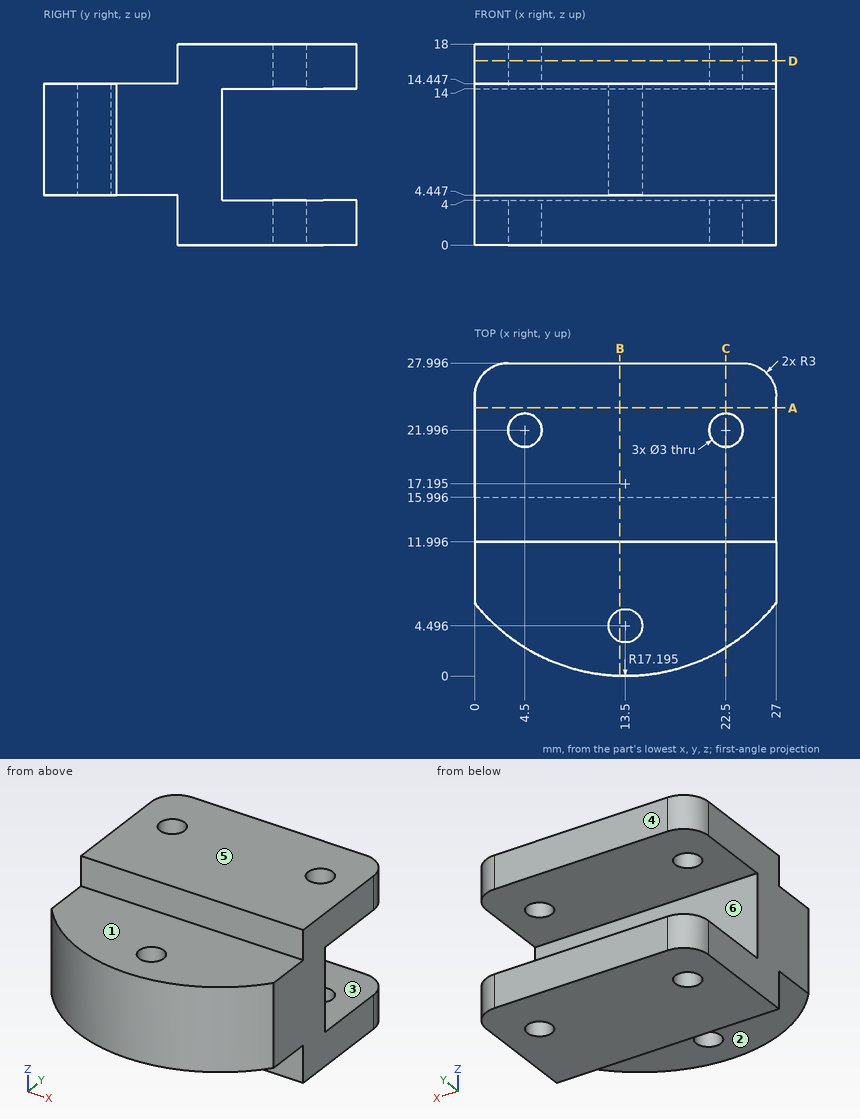
Job drawing, mm, ordinate dimensions from the low corner. One solid piece. A direction names the side the tool comes from. Coordinates: 2 decimals unless noted, no trailing zeros. Write each loop counter-clockwise with the first axis right and the second up, starting at its lowest first coordinate (ties: lowest second). Pieces come first, ordered by that corner, then holes. Notation, with made-up numbers: (15, -8) -> (49, -8) arc R14 cw to (49, 17) -> close; hole circle Ø6 at (50, 32.25). An arc over 180 degrees is marked (long way). Use CSV: the item, a comma, the result in double quotes. Start each with the question number.
Item 1: Band-saw the part on D-D, the plane z = 16.5. Write the cut outline in (x, y).
Item 2: Drop flat-ended pins along their axis: P1, Ø4, axis at y = 4.5, z = 8.5, coming from the +X side (1 decimal); P2, Ø5, axis at x = 4.5, y = 22, coming from the +Z side; P3, Ø1.8, axis at x = 7, z = 16, coming from the -Y side; P4, Ø6, axis at x = 13.5, y = 7.5, coming from the -Z side. Give the stop position or say it passes through.
Item 3: Band-saw the part on A-A, the plane y = 24. Write the cut outline in (x, z).
Item 4: Wall check: probe 1 along Z at (x, y) = (15.5, 22); probe 2 along Y at (x, z) = (22.5, 2); probe 3 along Y at (x, z) = (13.5, 11). Give the ranges that are in metal, low to high.
Item 5: Two-plate mould, pull along Z, no slides. Class the marked faces 4, 5 and 6: +Z half, -Z half, draft (parallel to the pull), parting line (faces both ways), or undercut.
Item 6: Tool access for the marked faces 1, 2 and 3: list every direction of +Z, -Z, +X, -X, +Y, -Y with a clear straight run to the whole face (end or side of a thin tool).
Item 7: Band-saw the part on B-B, the plane x = 13. Write the cut outline in (y, z).
Item 8: Band-saw the part on C-C, the plane x = 22.5. Write the cut outline in (y, z).
Response values:
1,outline,"(0, 12) -> (27, 12) -> (27, 25) arc R3 ccw to (24, 28) -> (3, 28) arc R3 ccw to (0, 25) -> close; hole circle Ø3 at (4.5, 22); hole circle Ø3 at (22.5, 22)"
2,P1,"stops at x = 27"
2,P2,"stops at z = 18"
2,P3,"stops at y = 12"
2,P4,"stops at z = 4.45"
3,outline,"(0, 0) -> (27, 0) -> (27, 4) -> (0, 4) -> close; (0, 14) -> (27, 14) -> (27, 18) -> (0, 18) -> close"
4,probe 1,"z = 0 to 4, 14 to 18"
4,probe 2,"y = 12 to 20.5, 23.5 to 28"
4,probe 3,"y = 0 to 3, 6 to 16"
5,face 4,"draft"
5,face 5,"+Z half"
5,face 6,"undercut"
6,face 1,"+Z, +X, -X, -Y"
6,face 2,"-Z, +X, -X, -Y"
6,face 3,"+X, -X, +Y"
7,outline,"(0.01, 4.45) -> (3.08, 4.45) -> (3.08, 14.45) -> (0.01, 14.45) -> close; (5.91, 4.45) -> (12, 4.45) -> (12, 0) -> (28, 0) -> (28, 4) -> (16, 4) -> (16, 14) -> (28, 14) -> (28, 18) -> (12, 18) -> (12, 14.45) -> (5.91, 14.45) -> close"
8,outline,"(2.54, 4.45) -> (12, 4.45) -> (12, 0) -> (20.5, 0) -> (20.5, 4) -> (16, 4) -> (16, 14) -> (20.5, 14) -> (20.5, 18) -> (12, 18) -> (12, 14.45) -> (2.54, 14.45) -> close; (23.5, 0) -> (28, 0) -> (28, 4) -> (23.5, 4) -> close; (23.5, 14) -> (28, 14) -> (28, 18) -> (23.5, 18) -> close"
